Read the model definition and answer for the solid it produces. Units are mm, in the model's axes. A direction names the side the tool comes from. Give positions to 0.01 mm unless a question says otherwise; leave off trailing zeros. Loops run counter-clockwise (first coordinate to the right, second up) from the corner with the lowest first, then second, coordinate; pieces in that order, holes last. Notation, with made-up numbers: (-26, -2) - (-21, -2) arc R19 ccw to (-21, 32) - close; hole circle Ø1 at (12.5, 37). An arc over 180 degrees is marked (long way). Use a Markdown table: item, result. Add a question column.
Item 1: A cutting plane is placed at B-B (y = 76.5). Determine the outline of the cut face in (x, z).
Item 2: Each of these flat-tipped pins is pushed along its axis until it touches: P1, Ø1, axis at y = 89, z = -7, coming from the -X side; P2, Ø2, axis at x = 67.5, y = 117.5, coming from the -Z side; P3, Ø4, axis at x = 161, z = -8, coming from the +Y side; P4, Ø5.5, axis at x = 43.5, z = -8.5, coming from the -Y side. Where does it stop, or does it pass through?
Item 3: Which of the six approach directions +Z, -Z, +X, -X, +Y, -Y give full straight-line access (tool end or side, diameter ignored) to faces 1 (the face through (32, 40, -8)), 2 (the face through (153, 24, -8)), 3 (the face through (48, 23, -8)), 4 (the face through (170, 114, -8)), 5 (the face through (33.085, 31.381, -15.342))?
Item 4: Consider probe 1 along Y at (x, z) = (166, -9); probe 2 along Y at (x, z) = (67.5, -9.2); probe 3 along X at (y, z) = (36, -11.75). Determine where each line is inside the solid, lowest interval first. Write a range as [from, to].
Item 5: For a pull along Y with two mould halves and no side action, classify faces 6 (the face through (153, 77, -8)), 7 (the face through (170, 33, -8)), 8 (the face through (31, 120, -8)), 9 (the face through (48, 129, -8)) as +Y half, -Y half, draft (parallel to the pull), parting line (faces both ways), or undercut.
Item 6: A cutting plane is placed at C-C (x = 100.5). Determine the outline of the cut face in (y, z), plus the area to 3 significant figures.
Item 7: A cutting plane is placed at A-A (z = -18). Give the number of separate pieces and of enclosed holes in the cut face, plus the area to 3 significant figures.
Autodesk Inventor part; units mm, degrees
ref_plane "YZ Plane" through (0, 0, 0) normal (1, 0, 0) x (0, 1, 0)
ref_plane "XZ Plane" through (0, 0, 0) normal (0, 1, 0) x (-1, 0, 0)
ref_plane "XY Plane" through (0, 0, 0) normal (0, 0, 1) x (1, 0, 0)
ref_plane "Arbeitsebene1" through (145, 129, -5.4115) normal (0, 0, -1) x (-1, 0, 0)
sketch "Skizze1" plane through (145, 129, -5.4115) normal (0, 0, -1) x (-1, 0, 0)
  line L0 (0, -105) -> (89, -105)
  line L1 (89, -105) -> (89, 0)
  line L2 (0, 0) -> (0, -105)
  line L3 (89, 0) -> (0, 0)
  line L4 (89, -105) -> (0, 0)
  line L5 (0, -105) -> (89, 0)
  line L6 (97, 8) -> (-8, 8)
  line L7 (-8, 8) -> (-8, -113)
  line L8 (-8, -113) -> (97, -113)
  line L9 (97, -113) -> (97, 8)
  line L10 (97, 8) -> (-8, -113) construction
  line L11 (-8, 8) -> (97, -113) construction
  point P0 (145, -129)
  point P1 (44.5, -52.5)
  dimension "d1" = 105
  dimension "d2" = 121
extrude "Extrusion1" add sketch "Skizze1" along normal blind 5 contours L5 L4 L0 | L2 L4 L5 | L4 L5 L1 | L3 L5 L4 | L9 L8 L7 L6
sketch "Skizze3" plane through (145, 129, -10.4115) normal (0, 0, -1) x (-1, 0, 0)
  circle A0 centre (10, -96.5) radius 1
  circle A1 centre (10, -11.5) radius 1
  circle A2 centre (77.5, -96.5) radius 1
  circle A3 centre (77.5, -11.5) radius 1
  circle A4 centre (77.5, -11.5) radius 4
  circle A5 centre (77.5, -11.5) radius 1.25
  circle A6 centre (77.5, -96.5) radius 4
  circle A7 centre (77.5, -96.5) radius 1.25
  circle A8 centre (10, -96.5) radius 1.25
  circle A9 centre (10, -11.5) radius 1.25
  point P0 (145, -129)
  dimension "d12" = 2.5
  dimension "d13" = 2.5
  dimension "d14" = 2.5
  dimension "d15" = 2.5
extrude "Extrusion3" cut sketch "Skizze3" against normal blind 25.25 contours A0 | A1 | A2 | A3 | A5 | A7 | A8 | A9
sketch "Skizze5" plane through (48, 16, -5.4115) normal (-1, 0, 0) x (0, 0, 1)
  line L0 (0, 0) -> (0, 121)
  line L1 (0, 121) -> (-5, 121)
  line L2 (-5, 0) -> (-5, 121)
  line L3 (0, 0) -> (-5, 0)
  line L4 (0, 121) -> (0, 106)
  line L5 (0, 0) -> (0, 15)
  line L6 (0, 106) -> (-5, 106)
  line L7 (-5, 106) -> (-5, 96)
  line L8 (-5, 96) -> (0, 96)
  line L9 (0, 96) -> (0, 106)
  line L10 (0, 15) -> (-5, 15)
  line L11 (-5, 15) -> (-5, 25)
  line L12 (-5, 25) -> (0, 25)
  line L13 (0, 25) -> (0, 15)
  point P0 (5.4115, -16)
  dimension "d24" = 15
  dimension "d25" = 15
  dimension "d26" = 10
  dimension "d27" = 10
extrude "Extrusion5" add sketch "Skizze5" along normal blind 18 contours L10 L2 L12 L0 | L8 L2 L6 L0
fillet "Rundung1" radius 5 4 edges at (30, 122, -7.9115) (30, 112, -7.9115) (30, 41, -7.9115) (30, 31, -7.9115)
sketch "Skizze6" plane through (153, 16, -5.4115) normal (1, 0, 0) x (0, 0, -1)
  line L0 (0, 121) -> (0, 0)
  line L1 (0, 0) -> (5, 0)
  line L2 (5, 121) -> (5, 0)
  line L3 (0, 121) -> (5, 121)
  line L4 (0, 0) -> (0, 15)
  line L5 (0, 0) -> (0, 15)
  line L6 (0, 121) -> (0, 106)
  line L7 (0, 15) -> (5, 15)
  line L8 (5, 15) -> (5, 25)
  line L9 (5, 25) -> (0, 25)
  line L10 (0, 25) -> (0, 15)
  line L11 (0, 96) -> (5, 96)
  line L12 (0, 106) -> (5, 106)
  line L13 (5, 106) -> (5, 96)
  line L14 (5, 96) -> (0, 96)
  line L15 (0, 96) -> (0, 106)
  point P0 (-5.4115, -16)
  dimension "d31" = 15
  dimension "d32" = 15
  dimension "d33" = 10
  dimension "d34" = 10
extrude "Extrusion6" add sketch "Skizze6" along normal blind 18 contours L12 L2 L11 L0 | L9 L2 L7 L0
fillet "Rundung2" radius 5 4 edges at (171, 112, -7.9115) (171, 122, -7.9115) (171, 31, -7.9115) (171, 41, -7.9115)
sketch "Skizze7" plane through (145, 129, -5.4115) normal (0, 0, 1) x (1, 0, 0)
  arc A0 (21, -98) -> (21, -88) centre (21, -93) ccw
  line L0 (8, -88) -> (21, -88)
  line L1 (8, -17) -> (8, -88)
  line L2 (8, -17) -> (21, -17)
  arc A1 (21, -17) -> (21, -7) centre (21, -12) ccw
  line L3 (8, -7) -> (21, -7)
  line L4 (8, 8) -> (8, -7)
  line L5 (-97, 8) -> (8, 8)
  line L6 (-97, -7) -> (-97, 8)
  line L7 (-97, -7) -> (-110, -7)
  arc A2 (-110, -7) -> (-110, -17) centre (-110, -12) ccw
  line L8 (-97, -17) -> (-110, -17)
  line L9 (-97, -88) -> (-97, -17)
  line L10 (-97, -88) -> (-110, -88)
  arc A3 (-110, -88) -> (-110, -98) centre (-110, -93) ccw
  line L11 (-97, -98) -> (-110, -98)
  line L12 (-97, -113) -> (-97, -98)
  line L13 (8, -113) -> (-97, -113)
  line L14 (8, -98) -> (8, -113)
  line L15 (8, -98) -> (21, -98)
  circle A4 centre (-110, -12) radius 2.1
  circle A5 centre (21, -12) radius 2.1
  circle A6 centre (21, -93) radius 2.1
  arc A7 (-110, -88) -> (-110, -98) centre (-110, -93) ccw
  circle A8 centre (-110, -93) radius 2.1
  point P0 (-145, -129)
  dimension "d38" = 4.2
  dimension "d39" = 4.2
  dimension "d40" = 4.2
  dimension "d41" = 4.2
extrude "Extrusion7" cut sketch "Skizze7" against normal blind 18 contours A4 | A5 | A6 | A8
sketch "Skizze8" plane through (145, 129, -10.4115) normal (0, 0, -1) x (-1, 0, 0)
  circle A0 centre (-21, -93) radius 2.1
  circle A1 centre (-21, -12) radius 2.1
  circle A2 centre (110, -93) radius 2.1
  circle A3 centre (110, -12) radius 2.1
  arc A4 (-21, -88) -> (-21, -98) centre (-21, -93) ccw
  line L0 (-8, -98) -> (-21, -98)
  line L1 (-8, -98) -> (-8, -113)
  line L2 (-8, -113) -> (97, -113)
  line L3 (97, -113) -> (97, -98)
  line L4 (97, -98) -> (110, -98)
  arc A5 (110, -98) -> (110, -88) centre (110, -93) ccw
  line L5 (97, -88) -> (110, -88)
  line L6 (97, -88) -> (97, -17)
  line L7 (97, -17) -> (110, -17)
  arc A6 (110, -17) -> (110, -7) centre (110, -12) ccw
  line L8 (97, -7) -> (110, -7)
  line L9 (97, -7) -> (97, 8)
  line L10 (97, 8) -> (-8, 8)
  line L11 (-8, 8) -> (-8, -7)
  line L12 (-8, -7) -> (-21, -7)
  arc A7 (-21, -7) -> (-21, -17) centre (-21, -12) ccw
  line L13 (-8, -17) -> (-21, -17)
  line L14 (-8, -17) -> (-8, -88)
  line L15 (-8, -88) -> (-21, -88)
  circle A8 centre (-21, -93) radius 5
  circle A9 centre (-21, -12) radius 5
  circle A10 centre (110, -12) radius 5
  circle A11 centre (110, -93) radius 5
  line L16 (97, -113) -> (-8, 8)
  circle A12 centre (44.5, -52.5) radius 10
  point P0 (145, -129)
  dimension "d44" = 20
extrude "Extrusion8" add sketch "Skizze8" along normal blind 10 contours A8 A4 | A7 A9 | A12 L16 | L16 A12 | A11 A5 | A6 A10
properties part number "PCB_Gehaeuse_o"
Geometry says:
| question | item | result |
|---|---|---|
| 1 | outline | (48, -10.41) - (90.5, -10.41) - (90.5, -20.41) - (110.5, -20.41) - (110.5, -10.41) - (153, -10.41) - (153, -5.41) - (48, -5.41) - close |
| 2 | P1 | x = 48 |
| 2 | P2 | through |
| 2 | P3 | y = 122 |
| 2 | P4 | y = 31 |
| 3 | face 1 | +Z, -Z, -X |
| 3 | face 2 | +Z, -Z, +X, -Y |
| 3 | face 3 | +Z, -Z, -X, -Y |
| 3 | face 4 | +Z, -Z, +X |
| 3 | face 5 | -Z |
| 4 | probe 1 | [31, 33.9], [38.1, 41], [112, 114.9], [119.1, 122] |
| 4 | probe 2 | [16, 31.25], [33.75, 116.25], [118.75, 137] |
| 4 | probe 3 | [30, 32.9], [37.1, 40], [161, 163.9], [168.1, 171] |
| 5 | face 6 | undercut |
| 5 | face 7 | -Y half |
| 5 | face 8 | +Y half |
| 5 | face 9 | draft |
| 6 | outline | (16, -10.41) - (66.5, -10.41) - (66.5, -20.41) - (86.5, -20.41) - (86.5, -10.41) - (137, -10.41) - (137, -5.41) - (16, -5.41) - close |
| 6 | area | 805 mm² |
| 7 | separate pieces | 5 |
| 7 | enclosed holes | 4 |
| 7 | area | 573 mm² |
